For this review, take the finished solid that the model builds, in its own axes (mm). A direction names the side the tool comes from. Coordinates: 2 decimals unless noted, no trailing zeros. Write each loop counter-clockwise with the first axis right and the second up, starting at its lowest first coordinate (ties: lowest second). Pieces come first, ordered by that corner, then holes.
```python
from build123d import *

# Parameters (mm, degrees)
SK_CHAIN_PROFILE_W = 12
SK_CHAIN_PROFILE_H = 5


with BuildPart() as part:
    # FT_Chain_Envelope: sweep along a path in SK_Chain_Path
    with BuildLine(Plane.XY) as ft_chain_envelope_path:
        Line((0.235356499, -27.424490106), (-299.74255, -29.998895305))
        ThreePointArc((-299.74255, -29.998895305), (-330, 0), (-299.74255, 29.998895305))
        Line((-299.74255, 29.998895305), (0.235356499, 27.424490106))
        ThreePointArc((0.235356499, 27.424490106), (27.4255, 0), (0.235356499, -27.424490106))
    # SK_Chain_Profile → FT_Chain_Envelope (sweep)
    with BuildSketch(Plane(origin=(-299.74255, 29.998895305, 0), x_dir=(0, 0, -1), z_dir=(0.9999631768206378, -0.008581666666666639, 0))):
        Rectangle(SK_CHAIN_PROFILE_W, SK_CHAIN_PROFILE_H)
    sweep(path=ft_chain_envelope_path.line)


solid = part.part
```
1) Clearance check with flat-ended pins moving along their axes: P1, Ø4, axis at y = -4.5, z = 3, coming from the +X side; P2, Ø3, axis at x = -115.5, z = -2, coming from the -Y side; P3, Ø3, axis at x = -80.5, z = -0.5, coming from the +Y side. State where each tip first meets the part, or that it passes through.
2) Consider section A-A (y = 0). Give the boundary of the cut face in (x, z), then the cut area to 3 significant figures.
3) Tool access review of faces 4 (the face through (-327.493, -0.608, -0.084)), 5 (the face through (-165, -28, 6)): name each direction out of +Z, -Z, +X, -X, +Y, -Y from which nothing blocks a thin tool from reaching the whole face with its end or side.
4) Consider section B-B (z = -4). Give the boundary of the cut face in (x, y), then the cut area to 3 significant figures.
5) Consider section C-C (x = -188). Give the boundary of the cut face in (y, z), then the cut area to 3 significant figures.
6) The part is to be moulded in two halves that separate along X. For faces 1 (the face through (24.92, 0.55, -0.08)), 2 (the face through (29.92, 0.65, 0.08)), 3 (the face through (-152, 28, -6)), say which applies: pulls with the +X half, pulls with the -X half, needs draft (parallel to the pull), parting line crosses it, or undercut.
7) For L1, parallel to X at y = -21, z = -4.25; L2, parallel to X at y = -20.5, z = -2.75; L3, parallel to Y at x = -43, z = -5, list the stretches that pass through material, from the lowest coordinate up.
Results:
1. P1: stops at x = 29.82
1. P2: stops at y = -30.93
1. P3: stops at y = 30.63
2. outline: (-332.5, -6) - (-327.5, -6) - (-327.5, 6) - (-332.5, 6) - close; (24.93, -6) - (29.93, -6) - (29.93, 6) - (24.93, 6) - close
2. area: 120 mm2
3. face 4: +Z, -Z
3. face 5: +Z, +X, -X, +Y, -Y
4. outline: (-299.72, -32.5) - (0.26, -29.92) arc R29.93 ccw to (0.26, 29.92) - (-299.72, 32.5) arc R32.5 ccw (long way) to start; hole (-299.76, -27.5) - (0.21, -24.92) arc R24.93 ccw to (0.21, 24.92) - (-299.76, 27.5) arc R27.5 ccw (long way) to start
4. area: 3,900 mm2
5. outline: (-31.54, -6) - (-26.54, -6) - (-26.54, 6) - (-31.54, 6) - close; (26.54, -6) - (31.54, -6) - (31.54, 6) - (26.54, 6) - close
5. area: 120 mm2
6. face 1: undercut
6. face 2: pulls with the +X half
6. face 3: needs draft
7. L1: x = -324.8 to -317.76, 13.43 to 21.32
7. L2: x = -325.22 to -318.33, 14.18 to 21.8
7. L3: y = -30.3 to -25.3, 25.3 to 30.3
